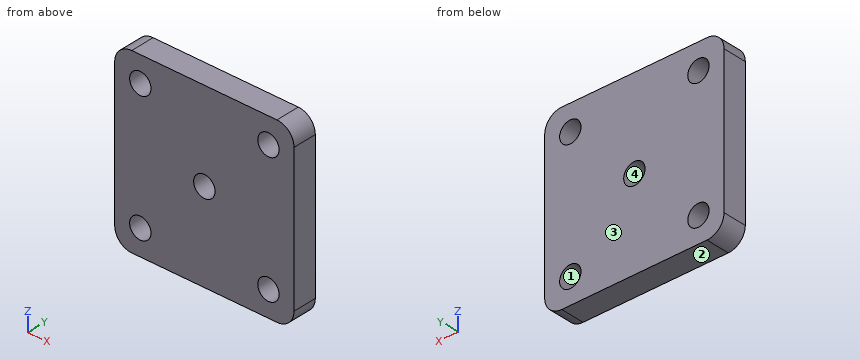
from build123d import *

# Parameters (mm, degrees)
F0_R     = 2.5
F1_DEPTH = 5.6


with BuildPart() as f1:
    # F0 (on Front) → F1 (new body)
    with BuildSketch(Plane.XZ):
        with BuildLine():
            ThreePointArc((21, 17), (19.828427, 19.828427), (17, 21))
            Line((17, 21), (-17, 21))
            ThreePointArc((-17, 21), (-19.828427, 19.828427), (-21, 17))
            Line((-21, 17), (-21, -17))
            ThreePointArc((-21, -17), (-19.828427, -19.828427), (-17, -21))
            Line((-17, -21), (17, -21))
            ThreePointArc((17, -21), (19.828427, -19.828427), (21, -17))
            Line((21, -17), (21, 17))
        make_face()
        with Locations((-15, -15)):
            Circle(F0_R, mode=Mode.SUBTRACT)
        with Locations((15, -15)):
            Circle(F0_R, mode=Mode.SUBTRACT)
        with Locations((-15, 15)):
            Circle(F0_R, mode=Mode.SUBTRACT)
        Circle(F0_R, mode=Mode.SUBTRACT)
        with Locations((15, 15)):
            Circle(F0_R, mode=Mode.SUBTRACT)
    extrude(amount=F1_DEPTH)


solid = f1.part
Check sheet for the modelled part. Datum: model origin and axes. Units: mm. Face numbers are marked on the shaded views. Give positions to 0.01 mm unless a question says otherwise; leave off trailing zeros. Order: outer loops, then holes, each group sorted by start corner. A loop starts at its lowest first (then second) coordinate and runs counter-clockwise, first axis right, second up. Notation, with made-up numbers: (-29.75, -1.75) - (-1.75, -1.75) arc R21 cw to (-1.75, 19.25) - close; hole circle Ø6 at (32.5, 57.5). An arc over 180 degrees is marked (long way). Answer as CSV lines item,"result".
1. Go/stop test with a flat-tipped pin: P1, Ø4.5, axis at x = 15, z = -15, coming from the -Y side. Record where the tip stops, or that it passes through.
Result sheet:
P1,"through"
2. Section check C-C (x = 0). Record the boundary of the cut face in (y, z).
Result sheet:
outline,"(-5.6, -21) - (0, -21) - (0, -2.5) - (-5.6, -2.5) - close; (-5.6, 2.5) - (0, 2.5) - (0, 21) - (-5.6, 21) - close"
3. Section check D-D (z = 15). Record the boundary of the cut face in (x, y), then the cut area to 3 significant figures.
Result sheet:
outline,"(-21, -5.6) - (-17.5, -5.6) - (-17.5, 0) - (-21, 0) - close; (-12.5, -5.6) - (12.5, -5.6) - (12.5, 0) - (-12.5, 0) - close; (17.5, -5.6) - (21, -5.6) - (21, 0) - (17.5, 0) - close"
area,"179 mm²"
4. Section check A-A (x = 16.5). Record the boundary of the cut face in (y, z), then the cut area to 3 significant figures.
Result sheet:
outline,"(-5.6, -21) - (0, -21) - (0, -17) - (-5.6, -17) - close; (-5.6, -13) - (0, -13) - (0, 13) - (-5.6, 13) - close; (-5.6, 17) - (0, 17) - (0, 21) - (-5.6, 21) - close"
area,"190 mm²"
5. Section check B-B (y = -1.25). Record the boundary of the cut face in (x, z), then the cut area to 3 significant figures.
Result sheet:
outline,"(-21, -17) arc R4 ccw to (-17, -21) - (17, -21) arc R4 ccw to (21, -17) - (21, 17) arc R4 ccw to (17, 21) - (-17, 21) arc R4 ccw to (-21, 17) - close; hole circle Ø5 at (-15, -15); hole circle Ø5 at (-15, 15); hole circle Ø5 at (0, 0); hole circle Ø5 at (15, -15); hole circle Ø5 at (15, 15)"
area,"1,650 mm²"
6. Scan lines: probe 1 along Z at (x, y) = (15, -1.6); probe 2 along Z at (x, y) = (0, -2.6); probe 3 along Z at (x, y) = (-13, -2.2). Record each from-to range of solid material in increasing order. Write a range as from..to.
Result sheet:
probe 1,"-21..-17.5, -12.5..12.5, 17.5..21"
probe 2,"-21..-2.5, 2.5..21"
probe 3,"-21..-16.5, -13.5..13.5, 16.5..21"
7. Mould release check, pull along Z, two halves, no side actions. Record for the marked faces 1, 2, 3 and 4: released by +Z, released by -Z, zero draft, split by the parting line, or undercut.
Result sheet:
face 1,"undercut"
face 2,"released by -Z"
face 3,"zero draft"
face 4,"undercut"
